Model file for the job. Use its own axes, mm. A direction names the side the tool comes from. Coordinates: 2 decimals unless noted, no trailing zeros. Write each loop counter-clockwise with the first axis right and the second up, starting at its lowest first coordinate (ties: lowest second). Pieces come first, ordered by that corner, then holes.
Q1. Band-saw the part on B-B, the plane x = 200.5. Write the cut outline in (y, z).
Q2. Pull direction Y, two halves, no side cores. Call faces 6 (the flat face through (203, 63.987, 1)), 7 (the cylindrical face through (208.386, 83.912, 1.479)), 8 (the flat face through (187.5, 86, 1)): released by +Y, released by -Y, zero draft, split by the parting line, or undercut.
Q3. Which spindle directions (+Z, -Z, +X, -X, +Y, -Y) get a long thin tool onto all of the face, cutting with end or side? Do faces 1 (the cylindrical face through (177.8, 64.94, 1.48)), 2 (the flat face through (203, 87.986, 1)), 3 (the flat face through (182.2, 76, 1)), 4 (the flat face through (187.5, 65, 1)), 5 (the flat face through (199.5, 87, 1)). Say none if no direction does.
Q4. Band-saw the part on C-C, the plane z = 1.65. Write the cut outline in (x, y), plus the area to 3 significant figures.
Q5. Drill centre lines: probe 1 along Y at (x, z) = (184.5, 1.85); probe 2 along Y at (x, z) = (193.5, 2.7); probe 3 along X at (y, z) = (79.75, 2.1). Where is each one in solid material? Low to high.
Q6. Band-saw the part on A-A, the plane y = 72. Write the cut outline in (x, z), plus the area to 3 significant figures.
Q7. Pin check, flat tips, straight feed: P1, Ø0.9, axis at y = 65, z = 1.5, coming from the -X side; P2, Ø1.5, axis at x = 181.5, y = 80.5, coming from the -Z side; P3, Ø0.9, axis at y = 66, z = 1, coming from the +X side; P4, Ø0.9, axis at y = 87, z = 1, coming from the +X side. Stop position of each tip, or through.
from build123d import *

# Parameters (mm, degrees)
SKETCH_1_R      = 1.500000002
SKETCH_1_R_2    = 1.5
SKETCH_1_R_3    = 1.500000008
EXTRUDE_1_DEPTH = 3


with BuildPart() as part:
    # 草圖1 → 填料-伸長1 (new body)
    with BuildSketch(Plane.XY):
        with BuildLine():
            Line((199.500112684, 87.98631657), (199.500112684, 84.98651657))
            Line((199.500112684, 84.98651657), (187.500112684, 84.98651657))
            Line((187.500112684, 84.98651657), (187.500112684, 87.98631657))
            Line((187.500112684, 87.98631657), (179.842912684, 87.98631657))
            ThreePointArc((179.842912684, 87.98631657), (177.823916024, 87.055493072), (177.000112684, 84.99051657))
            Line((177.000112684, 84.99051657), (177.000112684, 66.98231657))
            ThreePointArc((177.000112684, 66.98231657), (177.823916024, 64.917340067), (179.842912684, 63.98651657))
            Line((179.842912684, 63.98651657), (187.500112684, 63.98651657))
            Line((187.500112684, 63.98651657), (187.500112684, 66.98651657))
            Line((187.500112684, 66.98651657), (199.500112684, 66.98651657))
            Line((199.500112684, 66.98651657), (199.500112684, 63.98651657))
            Line((199.500112684, 63.98651657), (207.000112684, 63.98651657))
            ThreePointArc((207.000112684, 63.98651657), (209.097709344, 64.885982101), (210.000112684, 66.98231657))
            Line((210.000112684, 66.98231657), (210.000112685, 84.99051657))
            ThreePointArc((210.000112685, 84.99051657), (209.176309345, 87.055493072), (207.157312685, 87.98631657))
            Line((207.157312685, 87.98631657), (199.500112684, 87.98631657))
        make_face()
        with Locations((179.800012686, 67.486516568)):
            Circle(SKETCH_1_R, mode=Mode.SUBTRACT)
        with Locations((179.800062678, 84.486566583)):
            Circle(SKETCH_1_R_2, mode=Mode.SUBTRACT)
        with Locations((207.00011268, 84.486516578)):
            Circle(SKETCH_1_R_3, mode=Mode.SUBTRACT)
        with Locations((207.000062688, 67.486466573)):
            Circle(SKETCH_1_R_2, mode=Mode.SUBTRACT)
        Polygon((205.000112684, 73.588516578), (205.000112684, 69.888516578), (182.200112684, 69.888516578), (182.200112684, 82.088516578), (205.000112684, 82.088516578), (205.000112684, 78.588516578), (206.500112684, 78.588516578), (206.500112684, 73.588516578), align=None, mode=Mode.SUBTRACT)
    extrude(amount=EXTRUDE_1_DEPTH)


solid = part.part
Answer sheet:
1. outline: (63.99, 0) - (69.89, 0) - (69.89, 3) - (63.99, 3) - close; (82.09, 0) - (87.99, 0) - (87.99, 3) - (82.09, 3) - close
2. face 6: released by -Y
2. face 7: undercut
2. face 8: zero draft
3. face 1: +Z, -Z, -X, -Y
3. face 2: +Z, -Z, +X, -X, +Y
3. face 3: +Z, -Z
3. face 4: +Z, -Z, -Y
3. face 5: +Z, -Z, +Y
4. outline: (177, 66.98) arc R3 ccw to (179.84, 63.99) - (187.5, 63.99) - (187.5, 66.99) - (199.5, 66.99) - (199.5, 63.99) - (207, 63.99) arc R3.08 ccw to (210, 66.98) - (210, 84.99) arc R3 ccw to (207.16, 87.99) - (199.5, 87.99) - (199.5, 84.99) - (187.5, 84.99) - (187.5, 87.99) - (179.84, 87.99) arc R3 ccw to (177, 84.99) - close; hole circle Ø3 at (179.8, 67.49); hole circle Ø3 at (179.8, 84.49); hole (182.2, 69.89) - (205, 69.89) - (205, 73.59) - (206.5, 73.59) - (206.5, 78.59) - (205, 78.59) - (205, 82.09) - (182.2, 82.09) - close; hole circle Ø3 at (207, 67.49); hole circle Ø3 at (207, 84.49)
4. area: 398 mm2
5. probe 1: y = 63.99 to 69.89, 82.09 to 87.99
5. probe 2: y = 66.99 to 69.89, 82.09 to 84.99
5. probe 3: x = 177 to 182.2, 205 to 210
6. outline: (177, 0) - (182.2, 0) - (182.2, 3) - (177, 3) - close; (205, 0) - (210, 0) - (210, 3) - (205, 3) - close
6. area: 30.6 mm2
7. P1: stops at x = 177.42
7. P2: stops at z = 0
7. P3: stops at x = 209.94
7. P4: stops at x = 209.56
